CAD build for the part. Positions are in the model's coordinates, mm. A direction names the side the tool comes from. Give positions to 0.01 mm unless a question says otherwise; leave off trailing zeros. Write each loop counter-clockwise with the first axis right and the second up, starting at its lowest first coordinate (ties: lowest second). Pieces come first, ordered by that corner, then holes. Notation, with made-up numbers: (71.5, -17) -> (90.5, -17) arc R30 ccw to (90.5, 14) -> close; hole circle Ø3 at (33.25, 21.25). An arc over 180 degrees is marked (long way). Use one line per item in the form item = value. Start each with the question number.
from build123d import *

# Parameters (mm, degrees)
BOSS_EXTRU_1_DEPTH      = 8
BOSS_EXTRU_2_DEPTH      = 15
CONG_1_R                = 20
CONG_2_R                = 4
ESQUISSE3_R             = 7.5
BOSS_EXTRU_3_DEPTH      = 8
ENL_V_MAT_EXTRU_1_DEPTH = 141.744449269


with BuildPart() as part:
    # Esquisse1 → Boss.-Extru.1 (new body)
    with BuildSketch(Plane.XY):
        Polygon((64, 0), (64, 50.343145751), (0, 114.343145751), (5.656854249, 120), (68, 57.656854249), (130.343145751, 120), (136, 114.343145751), (72, 50.343145751), (72, 0), align=None)
    extrude(amount=BOSS_EXTRU_1_DEPTH)

    # Esquisse2 → Boss.-Extru.2 (add)
    with BuildSketch(Plane(origin=(0, 0, 0), x_dir=(-1, 0, 0), z_dir=(0, 0, -1))):
        Polygon((-130.343145751, 108.686291501), (-136, 114.343145751), (-130.343145751, 120), (-124.686291501, 114.343145751), align=None)
        Polygon((0, 114.343145751), (-5.656854249, 108.686291501), (-11.313708499, 114.343145751), (-5.656854249, 120), align=None)
    extrude(amount=BOSS_EXTRU_2_DEPTH)

    # Congé1
    cong_1_edges = [part.edges().sort_by_distance(p)[0] for p in [
        (64, 50.343145751, 4),
        (68, 57.656854249, 4),
        (72, 50.343145751, 4),
    ]]
    fillet(cong_1_edges, radius=CONG_1_R)

    # Congé2
    cong_2_edges = [part.edges().sort_by_distance(p)[0] for p in [
        (133.171572875, 117.171572875, 8),
        (2.828427125, 117.171572875, 8),
    ]]
    fillet(cong_2_edges, radius=CONG_2_R)

    # Esquisse3 → Boss.-Extru.3 (add)
    with BuildSketch(Plane.ZY.offset(-64)):
        with Locations((4, 0)):
            Circle(ESQUISSE3_R)
    extrude(amount=-BOSS_EXTRU_3_DEPTH)

    # Esquisse4 → Enlèv. mat.-Extru.1 (cut, through all)
    with BuildSketch(Plane.ZY.offset(-64)):
        with BuildLine():
            Line((2.5, 3.708099244), (2.5, 6))
            Line((2.5, 6), (5.5, 6))
            Line((5.5, 6), (5.5, 3.708099244))
            ThreePointArc((5.5, 3.708099244), (4, -4), (2.5, 3.708099244))
        make_face()
    extrude(amount=-ENL_V_MAT_EXTRU_1_DEPTH, mode=Mode.SUBTRACT)


solid = part.part
1) Cut at B-B (y = 0). Give the cut face in (x, z), and give its area (3 significant figures).
2) Two-plate mould, pull along Z, no slides. Class faces 4 (the face through (68, -4, 4)), 5 (the face through (72, 18, 4)), 6 (the face through (68, 65, 0)): released by +Z, released by -Z, zero draft, split by the parting line, or undercut.
3) 3-axis set-ups, long thin cutter, end or side, ignore diameter. For faces 1 (the face through (8.45, 111.48, -7.4)), 2 (the face through (68, 6, 4)), 3 (the face through (73, 66, 8)): which of +Z, -Z, +X, -X, +Y, -Y reach the whole face in a straight line?
4) Cut at A-A (z = -5.25). Give the cut face in (x, y), and give its area (3 significant figures).
5) Pin check, flat tips, straight feed: pin 1 (5 mm diameter, centred on x = 25, z = -1.5, fed in from +Y); pin 2 (1 mm diameter, centred on x = 106, z = 3.5, fed in from -Y); pin 3 (2.5 mm diameter, centred on x = 67, y = 5, fed in from +Z). Stop position of each tip, or through.
6) Wall check: line 1 along Z through (x, y) = (69.25, 0); line 2 along Y through (x, z) = (68.5, 4); line 3 along Y through (x, z) = (69.5, 4). Give the ranges that are in metal, low to high. Write a range as from..to.
7) Cut at C-C (x = 36.5). Give the cut face in (y, z).
Final values:
q1.outline = (64, -3.5) -> (72, -3.5) -> (72, 0) -> (64, 0) -> close; (64, 8) -> (72, 8) -> (72, 11.5) -> (64, 11.5) -> close
q1.area = 56.0 mm^2
q2.face_4 = undercut
q2.face_5 = zero draft
q2.face_6 = released by -Z
q3.face_1 = -Z, -Y
q3.face_2 = +X, -X
q3.face_3 = +Z, +X, -X, +Y
q4.outline = (0, 114.34) -> (5.66, 108.69) -> (11.31, 114.34) -> (5.66, 120) -> close; (124.69, 114.34) -> (130.34, 108.69) -> (136, 114.34) -> (130.34, 120) -> close
q4.area = 128 mm^2
q5.pin_1 = 102.66
q5.pin_2 = 83.84
q5.pin_3 = 10.5
q6.line_1 = -3.5..0, 8..11.5
q6.line_2 = -7.5..-4, 6..65.95
q6.line_3 = -7.5..-4, 6..66
q7.outline = (77.84, 0) -> (89.16, 0) -> (89.16, 8) -> (77.84, 8) -> close
